from build123d import *

# Parameters (mm, degrees)
SKETCH103_W             = 21
SKETCH103_H             = 19
EXTRUDE095_DEPTH        = 2
SKETCH127_R             = 1.6
EXTRUDE117_DEPTH        = 10
BODY090_PLACEMENT_ANGLE = 90
BODY091_PLACEMENT_ANGLE = 90
BODY092_PLACEMENT_ANGLE = 90
BODY093_PLACEMENT_ANGLE = 90
SKETCH135_W             = 33
SKETCH135_H             = 7.5
EXTRUDE125_DEPTH        = 4
SKETCH102_W             = 126
SKETCH102_H             = 18
SKETCH102_W_2           = 80
SKETCH102_H_2           = 14
SKETCH102_W_3           = 77
SKETCH102_H_3           = 12
EXTRUDE094_DEPTH        = 4
EXTRUDE077_DEPTH        = 12.5


with BuildPart() as extrude095:
    # Sketch103 → Extrude095 (new body)
    with BuildSketch(Plane.XZ.offset(0.5)):
        with Locations((153, -16.5)):
            Rectangle(SKETCH103_W, SKETCH103_H)
    extrude(amount=-EXTRUDE095_DEPTH)


with BuildPart() as screw_outer:
    # Sketch127 → Extrude117 (new body)
    with BuildSketch(Plane.XY):
        Circle(SKETCH127_R)
    extrude(amount=EXTRUDE117_DEPTH)


with BuildPart() as screw_outer011:
    # Body090 base: copy of screw outer
    add(screw_outer.part)


with BuildPart() as screw_outer011_1:
    # Body090 placement: moved
    add(screw_outer011.part.moved(Location((-3.5, 88, -21))).rotate(Axis((-3.5, 88, -21), (0, 1, 0)), BODY090_PLACEMENT_ANGLE))


with BuildPart() as screw_outer012:
    # Body091 base: copy of screw outer
    add(screw_outer.part)


with BuildPart() as screw_outer012_1:
    # Body091 placement: moved
    add(screw_outer012.part.moved(Location((361.5, 88, -21))).rotate(Axis((361.5, 88, -21), (0, -1, 0)), BODY091_PLACEMENT_ANGLE))


with BuildPart() as screw_outer013:
    # Body092 base: copy of screw outer
    add(screw_outer.part)


with BuildPart() as screw_outer013_1:
    # Body092 placement: moved
    add(screw_outer013.part.moved(Location((133, -2.5, -21))).rotate(Axis((133, -2.5, -21), (-1, 0, 0)), BODY092_PLACEMENT_ANGLE))


with BuildPart() as screw_outer014:
    # Body093 base: copy of screw outer
    add(screw_outer.part)


with BuildPart() as screw_outer014_1:
    # Body093 placement: moved
    add(screw_outer014.part.moved(Location((260, -2.5, -21))).rotate(Axis((260, -2.5, -21), (-1, 0, 0)), BODY093_PLACEMENT_ANGLE))


with BuildPart() as power_cover001:
    # Sketch135 → Extrude125 (new body)
    with BuildSketch(Plane(origin=(-3.5, 0, 0), x_dir=(0, -1, 0), z_dir=(-1, 0, 0))):
        with Locations((-28, -15.75)):
            Rectangle(SKETCH135_W, SKETCH135_H)
    extrude(amount=-EXTRUDE125_DEPTH)


with BuildPart() as compound021:
    # Sketch102 → Extrude094 (new body)
    with BuildSketch(Plane.XZ.offset(3)):
        with Locations((59, -10)):
            Rectangle(SKETCH102_W, SKETCH102_H)
        with Locations((212, -9)):
            Rectangle(SKETCH102_W_2, SKETCH102_H_2)
        with Locations((306.93, -8)):
            Rectangle(SKETCH102_W_3, SKETCH102_H_3)
    extrude(amount=-EXTRUDE094_DEPTH)

    # Compound021: union Extrude095, screw outer011, screw outer012, screw outer013, screw outer014, power cover001
    add(extrude095.part)
    add(screw_outer011_1.part)
    add(screw_outer012_1.part)
    add(screw_outer013_1.part)
    add(screw_outer014_1.part)
    add(power_cover001.part)


with BuildPart() as side001:
    # Sketch085 → Extrude077 (new body)
    with BuildSketch(Plane(origin=(0, 0, -25), x_dir=(1, 0, 0), z_dir=(0, 0, -1))):
        Polygon((-2.5, 1.5), (360.5, 1.5), (360.5, -96.5), (358.5, -96.5), (358.5, -0.5), (-0.5, -0.5), (-0.5, -98), (-2.5, -98), align=None)
    extrude(amount=-EXTRUDE077_DEPTH)

    # Cut011: cut Compound021
    add(compound021.part, mode=Mode.SUBTRACT)


solid = side001.part
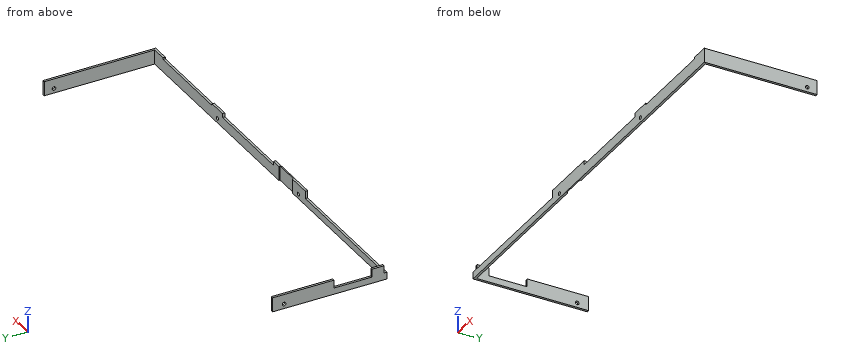
Here's how the part is built. I have some questions about the finished solid (model axes, mm). Round coordinates to 2 decimals unless told otherwise and drop trailing zeros. Write each loop counter-clockwise with the first axis right and the second up, starting at its lowest first coordinate (ties: lowest second). Pieces come first, ordered by that corner, then holes.
1. I need wall thicknesses on L1, parallel to X at y = 7, z = -22; L2, parallel to Z at x = 359.5, y = 88; L3, parallel to Y at x = -1.5, z = -21. Which ranges of each line are inside material? Lowest first, please.
2. Suppose I cut it at A-A (y = 52). List the corners of the cut face in (x, z) for me.
3. Suppose I cut it at C-C (x = 102.5). List the corners of the cut face in (y, z) for me, and give its area (3 significant figures).
4. Suppose I cut it at B-B (x = 221). List the corners of the cut face in (y, z) for me, and give its area (3 significant figures).
5. Will these pins go through, and if not, where does the flat tip stop? pin 1 Ø2 at (x, y) = (314.5, -0.5) entering from +Z; pin 2 Ø4 at (x, z) = (247.5, -19) entering from +Y; pin 3 Ø1 at (x, z) = (359.5, -17.5) entering from +Y.
Answer sheet:
1. L1: x = -2.5 to -0.5, 358.5 to 360.5
1. L2: z = -25 to -22.6, -19.4 to -12.5
1. L3: y = -1.5 to 86.4, 89.6 to 98
2. outline: (-2.5, -25) - (-0.5, -25) - (-0.5, -12.5) - (-2.5, -12.5) - close; (358.5, -25) - (360.5, -25) - (360.5, -12.5) - (358.5, -12.5) - close
3. outline: (-1.5, -25) - (0.5, -25) - (0.5, -19) - (-1.5, -19) - close
3. area: 12.0 mm2
4. outline: (-1.5, -25) - (0.5, -25) - (0.5, -16) - (-1.5, -16) - close
4. area: 18.0 mm2
5. pin 1: stops at z = -14
5. pin 2: stops at y = 0.5
5. pin 3: stops at y = 96.5
